Autodesk Inventor part; units mm, degrees
ref_plane "YZ Plane" through (0, 0, 0) normal (1, 0, 0) x (0, 1, 0)
ref_plane "XZ Plane" through (0, 0, 0) normal (0, 1, 0) x (-1, 0, 0)
ref_plane "XY Plane" through (0, 0, 0) normal (0, 0, 1) x (1, 0, 0)
sketch "Sketch1" plane through (0, 0, 0) normal (0, 0, 1) x (1, 0, 0)
  line L0 (1.5, 0) -> (1.5, 20)
  line L1 (-1.5, 20) -> (-1.5, 1.5)
  line L2 (1.5, 0) -> (1.5, -20)
  line L3 (-1.5, -20) -> (-1.5, -1.5)
  circle A0 centre (0, 20) radius 0.5
  arc A1 (1.5, 20) -> (-1.5, 20) centre (0, 20) ccw
  circle A2 centre (0, -20) radius 0.5
  arc A3 (-1.5, -20) -> (1.5, -20) centre (0, -20) ccw
  line L4 (-1.5, 1.5) -> (-1.5, -1.5)
  point P0 (0, 0)
extrude "Extrusion1" add sketch "Sketch1" along normal blind 9
sketch "Sketch3" plane through (-1.5, -20, 0) normal (-1, 0, 0) x (0, 0, 1)
  line L0 (9, 0) -> (9, 40)
  line L1 (9, 20) -> (0, 20)
  line L2 (0, 0) -> (0, 40)
  line L3 (9.5, 15) -> (-0.5, 15)
  line L4 (-0.5, 15) -> (-0.5, 25)
  line L5 (-0.5, 25) -> (9.5, 25)
  line L6 (9.5, 25) -> (9.5, 15)
  line L7 (9.5, 15) -> (-0.5, 25) construction
  line L8 (-0.5, 15) -> (9.5, 25) construction
  point P0 (4.5, 20)
  dimension "d29" = 10
  dimension "d30" = 10
extrude "Extrusion2" add sketch "Sketch3" along normal blind 53 and the other way blind 3
sketch "Sketch5" plane through (-54.5, -20, 0) normal (-1, 0, 0) x (0, 0, 1)
  line L0 (0, 15) -> (-0.5, 15) construction
  line L1 (9.5, 25) -> (9.5, 15) construction
  line L2 (-0.5, 15) -> (9.5, 25) construction
  point P0 (0, 20)
  point P1 (4.5, 20)
hole "Hole2" at (-54.5, 0, 4.5) direction (1, 0, 0) diameter 9 depth 16
sketch "Sketch6" plane through (1.5, 20, 9) normal (1, 0, 0) x (0, 0, -1)
  line L0 (9, -20) -> (-0.0817, -20) construction
  line L1 (6, -37.5) -> (6, -41.5)
  line L2 (6, -37.5) -> (3, -37.5)
  line L3 (3, -37.5) -> (3, -41.5)
  line L4 (6, -41.5) -> (3, -41.5)
  line L5 (6, -2.5) -> (6, 1.5)
  line L6 (6, -2.5) -> (3, -2.5)
  line L7 (3, -2.5) -> (3, 1.5)
  line L8 (6, 1.5) -> (3, 1.5)
extrude "Extrusion3" cut sketch "Sketch6" against normal through all
properties part number "Ciągaczka" material "Stainless Steel, 440C"
Geometry check sheet. Reference: the model listing, model coordinates, mm. A direction names the side the tool comes from. Give positions to 0.01 mm unless a question says otherwise; leave off trailing zeros. Loops run counter-clockwise (first coordinate to the right, second up) from the corner with the lowest first, then second, coordinate; pieces in that order, holes last. Notation, with made-up numbers: M -3,-28.5 L 15,-28.5 A22 cw 15,-11.5 Z; hole C 89.5,0.5 d3. An arc over 180 degrees is marked long. Write item = value, one per line. Start each with the question number.
1. Section check B-B, the plane z = 8. Enter the section's corners in (x, y), plus the area to 3 significant figures.
2. Thickness scan on probe 1 along Y at (x, z) = (0, 7.8); probe 2 along Y at (x, z) = (-46.75, 4.5); probe 3 along X at (y, z) = (20, 6.95). Record the ranges inside material, lowest first.
3. Section check A-A, the plane x = -48.5. Enter the section's corners in (y, z), plus the area to 3 significant figures.
4. Go/stop test with flat-tipped pins: P1, Ø3, axis at y = -7.5, z = 4.5, coming from the -X side; P2, Ø2.5, axis at x = 0.5, y = 19, coming from the -Z side; P3, Ø1.5, axis at x = -21, z = 3.5, coming from the +Y side. Record where each tip stops, or that it passes through.
5. Section check C-C, the plane y = 0. Enter the section's corners in (x, z), plus the area to 3 significant figures.
6. Section check D-D, the plane z = 4.5. Enter the section's corners in (x, y).
7. Tool access check on faces 1 (the face through (-1.5, 13, 4)), 2 (the face through (0, -19, 3)), 3 (the face through (0, -13, 9)). Record the directions out of +Z, -Z, +X, -X, +Y, -Y that give a thin tool (end or side, any length) a straight path to the whole face; none if there is none.
8. Draft check along Y on faces 4 (the face through (-38.5, 0, 4)), 5 (the face through (0, 13, 0)), 6 (the face through (0, 17.5, 4)). Enter one of: +Y half, -Y half, draft (parallel to the pull), parting line (faces both ways), or undercut.
Values follow:
q1.outline = M -54.5,-5 L -1.5,-5 L -1.5,-20 A1.5 ccw 1.5,-20 L 1.5,20 A1.5 ccw -1.5,20 L -1.5,5 L -54.5,5 L -54.5,2.83 L -38.5,2.83 L -38.5,-2.83 L -54.5,-2.83 Z; hole C 0,-20 d1; hole C 0,20 d1
q1.area = 565 mm^2
q2.probe_1 = -21.5 to -20.5, -19.5 to 19.5, 20.5 to 21.5
q2.probe_2 = -5 to -4.5, 4.5 to 5
q2.probe_3 = -1.5 to -0.5, 0.5 to 1.5
q3.outline = M -5,-0.5 L 5,-0.5 L 5,9.5 L -5,9.5 Z; hole C 0,4.5 d9
q3.area = 36.4 mm^2
q4.P1 = -1.5
q4.P2 = 0
q4.P3 = 5
q5.outline = M -54.5,-0.5 L 1.5,-0.5 L 1.5,9.5 L -54.5,9.5 L -54.5,9 L -38.5,9 L -38.5,0 L -54.5,0 Z
q5.area = 416 mm^2
q6.outline = M -54.5,-5 L -1.5,-5 L -1.5,-17.5 L 1.5,-17.5 L 1.5,17.5 L -1.5,17.5 L -1.5,5 L -54.5,5 L -54.5,4.5 L -38.5,4.5 L -38.5,-4.5 L -54.5,-4.5 Z
q7.face_1 = +Z, -Z, -X, +Y
q7.face_2 = +X, -X, -Y
q7.face_3 = +Z, +X, -X, -Y
q8.face_4 = undercut
q8.face_5 = draft
q8.face_6 = +Y half
